Autodesk Inventor part; units mm, degrees
ref_plane "YZ Plane" through (0, 0, 0) normal (1, 0, 0) x (0, 1, 0)
ref_plane "XZ Plane" through (0, 0, 0) normal (0, 1, 0) x (-1, 0, 0)
ref_plane "XY Plane" through (0, 0, 0) normal (0, 0, 1) x (1, 0, 0)
sketch "Sketch1" plane through (0, 0, 0) normal (0, 1, 0) x (-1, 0, 0)
  circle A0 centre (0, 0) radius 3.15
  line L0 (10, 5) -> (10, 30)
  line L1 (10, 30) -> (-10, 30)
  line L2 (-10, 30) -> (-10, 5)
  line L3 (10, -5) -> (10, -30)
  line L4 (10, -30) -> (-10, -30)
  line L5 (-10, -30) -> (-10, -5)
  line L6 (-10, 30) -> (-10, 15)
  line L7 (10, 30) -> (10, 15)
  line L8 (10, -30) -> (10, -15)
  line L9 (-10, -15) -> (-10, -30)
  line L10 (2.5151, -1.8965) -> (-2.5151, -1.8965)
  circle A1 centre (0, 0) radius 4.5
  line L11 (10, 0) -> (3.15, 0)
  line L12 (-3.15, 0) -> (-10, 0)
  line L13 (-10, 0) -> (-20, 0)
  line L14 (-20, 0) -> (-20, -5)
  line L15 (-20, -5) -> (-10, -5)
  line L16 (10, 0) -> (20, 0)
  line L17 (20, 0) -> (20, -5)
  line L18 (20, -5) -> (10, -5)
  line L19 (-4.5, 0) -> (-3.15, 0)
  line L20 (3.15, 0) -> (4.5, 0)
  line L21 (20, 0) -> (20, 5)
  line L22 (20, 5) -> (10, 5)
  line L23 (-20, 0) -> (-20, 5)
  line L24 (-20, 5) -> (-10, 5)
  circle A2 centre (-5, 22.5) radius 2.25
  circle A3 centre (6, 22.5) radius 2.25
  circle A4 centre (-6, -22.5) radius 2.25
  circle A5 centre (6, -22.5) radius 2.25
  circle A6 centre (-5, 22.5) radius 2.4
  circle A7 centre (6, 22.5) radius 2.4
  dimension "d0" = 6.3
  dimension "d6" = 15
  dimension "d34" = 9
  dimension "d35" = 10
  dimension "d36" = 5
  dimension "d37" = 10
  dimension "d38" = 5
  dimension "d43" = 5
  dimension "d44" = 5
  dimension "d45" = 4.5
  dimension "d46" = 4.5
  dimension "d47" = 4.5
  dimension "d48" = 4.5
  dimension "d61" = 4.8
  dimension "d62" = 4.8
extrude "Extrusion10" add sketch "Sketch1" along normal blind 10 contours A0 L12 A1 L11 | A1 L12 L13 L23 L24 L2 L1 L0 L22 L21 L16 L11 | A6 | A7 picked at (-4.0064, 0.359)
extrude "Extrusion11" add sketch "Sketch1" against normal blind 5 contours A0 L12 A1 L11 picked at (-4.0064, 0.359)
sketch "Sketch3" plane through (-3.15, 10, 0) normal (0, 0, -1) x (-1, 0, 0)
  line L0 (-23.15, -10) -> (-23.15, -5)
  line L1 (-23.15, -10) -> (-23.15, 0)
  line L2 (-23.15, -5) -> (-18.15, -5)
  line L3 (16.85, -10) -> (16.85, -5)
  line L4 (16.85, -10) -> (16.85, 0)
  line L5 (16.85, -5) -> (11.85, -5)
  circle A0 centre (-18.15, -5) radius 2.35
  circle A1 centre (11.85, -5) radius 2.35
  circle A2 centre (-18.15, -5) radius 2.4
  circle A3 centre (11.85, -5) radius 2.4
  point P0 (-3.15, -10)
  dimension "d53" = 5
  dimension "d54" = 5
  dimension "d55" = 5
  dimension "d56" = 5
  dimension "d57" = 4.7
  dimension "d58" = 4.7
  dimension "d65" = 4.8
  dimension "d66" = 4.8
extrude "Extrusion13" cut sketch "Sketch1" along normal blind 10 contours A6 | A7
extrude "Extrusion14" cut sketch "Sketch3" against normal blind 10 contours A0 | A2 | A1 | A3
properties part number "clip_to_shaft_holder(2)"
Here's how the part is built. I have some questions about the finished solid (model axes, mm). A direction names the side the tool comes from. Give positions to 0.01 mm unless a question says otherwise; leave off trailing zeros. Loops run counter-clockwise (first coordinate to the right, second up) from the corner with the lowest first, then second, coordinate; pieces in that order, holes last. Notation, with made-up numbers: M 37.25,82.25 L 57.25,82.25 A10 ccw 57.25,86.25 Z; hole C 40.5,54 d2. An arc over 180 degrees is marked long. Return JSON: item names as keys, results as strings.
Item 1: Imagine slicing it at B-B on z = 22.5. List the corners of the cut face in (x, y) for me.
A:
{"outline": "M -10,0 L -8.4,0 L -8.4,10 L -10,10 Z; M -3.6,0 L 2.6,0 L 2.6,10 L -3.6,10 Z; M 7.4,0 L 10,0 L 10,10 L 7.4,10 Z"}
Item 2: Imagine slicing it at C-C on x = 5. List the corners of the cut face in (y, z) for me, then the cut area to 3 significant figures.
A:
{"outline": "M 0,0 L 10,0 L 10,20.1 L 0,20.1 Z; M 0,24.9 L 10,24.9 L 10,30 L 0,30 Z", "area": "252 mm^2"}
Item 3: Please list where these lines run through material, in increasing order: line 1 (Z direction, x = -6, y = 6.75); line 2 (Y direction, x = 15, z = 2.4); line 3 (Y direction, x = -4.5, z = 19).
A:
{"line 1": "z = 0 to 20.1, 24.9 to 30", "line 2": "y = 0 to 2.6, 7.4 to 10", "line 3": "y = 0 to 10"}
Item 4: I'm going to push flat-ended pins straight in: pin 1 Ø1.5 at (x, y) = (-0.5, -1) entering from -Z; pin 2 Ø1 at (x, z) = (-11, 22) entering from -Y; pin 3 Ø8 at (y, z) = (2.5, 13) entering from -X; pin 4 Ø5 at (x, y) = (-16, 7) entering from +Z. Where does each tip first touch, or does it pass through?
A:
{"pin 1": "stops at z = 2.89", "pin 2": "passes through", "pin 3": "stops at x = -10", "pin 4": "stops at z = 5"}
Item 5: Thinking about a two-plate mould opening in X: for faces 1 (the flat face through (-17.3, 3.8, 5)), 2 (the cylindrical face through (-0.07, 2.61, 3.15)), 3 (the cylindrical face through (-0.1, -2.5, 4.5)), which applies, released by +X, released by -X, zero draft, split by the parting line, or undercut?
A:
{"face 1": "zero draft", "face 2": "undercut", "face 3": "split by the parting line"}
Item 6: Imagine slicing it at A-A on y = 5. List the corners of the cut face in (x, z) for me, then the cut area to 3 significant figures.
A:
{"outline": "M -20,0 L -17.4,0 L -17.4,5 L -20,5 Z; M -12.6,0 L -3.15,0 A3.15 cw 3.15,0 L 12.6,0 L 12.6,5 L 10,5 L 10,30 L -10,30 L -10,5 L -12.6,5 Z; M 17.4,0 L 20,0 L 20,5 L 17.4,5 Z; hole C -6,22.5 d4.8; hole C 5,22.5 d4.8", "area": "600 mm^2"}
Item 7: Imagine slicing it at D-D on y = 1.5. List the corners of the cut face in (x, z) for me, then the cut area to 3 significant figures.
A:
{"outline": "M -20,0 L -3.15,0 A3.15 cw 3.15,0 L 20,0 L 20,5 L 10,5 L 10,30 L -10,30 L -10,5 L -20,5 Z; hole C -6,22.5 d4.8; hole C 5,22.5 d4.8", "area": "648 mm^2"}
Item 8: On a 3-axis mill with a long thin cutter (end or side, diameter ignored), from which of +Z, -Z, +X, -X, +Y, -Y can I reach the whole of each face in a straight line? I mean faces 4 (the flat face through (-10, 5, 17)), 5 (the flat face through (17.3, 3.8, 5)), 6 (the cylindrical face through (17.398, 5.106, 2.465)). Say none if no direction works.
A:
{"face 4": "+Z, -X, +Y, -Y", "face 5": "+Z, +X, +Y, -Y", "face 6": "+Z, -Z"}
